from build123d import *

# Parameters (mm, degrees)
SKETCH2_W           = 508
SKETCH2_H           = 965.2
BOSS_EXTRUDE1_DEPTH = 152.4
FILLET1_R           = 15.24
FILLET2_R           = 15.24
SKETCH5_R           = 50.8
CUT_EXTRUDE1_DEPTH  = 718.072186045


with BuildPart() as part:
    # Sketch2 → Boss-Extrude1 (new body)
    with BuildSketch(Plane(origin=(0, 0, 0), x_dir=(1, 0, 0), z_dir=(0, 1, 0))):
        Rectangle(SKETCH2_W, SKETCH2_H)
    extrude(amount=BOSS_EXTRUDE1_DEPTH)

    # Fillet1
    fillet1_edges = [part.edges().sort_by_distance(p)[0] for p in [
        (-254, 152.4, 0),
        (0, 152.4, 482.6),
        (254, 152.4, 0),
        (0, 152.4, -482.6),
    ]]
    fillet(fillet1_edges, radius=FILLET1_R)

    # Fillet2
    # the kernel refuses this fillet: 15.24 mm, written as the material it takes off along each edge
    with BuildSketch(Plane(origin=(238.76, 137.16, -467.36), x_dir=(1, 0, 0), z_dir=(0, 0, -1))) as fillet2_piece_1_section:
        Polygon((0, 0), (FILLET2_R, 0), (FILLET2_R, -FILLET2_R), (0, -FILLET2_R), align=None)
    fillet2_piece_1 = extrude(amount=FILLET2_R, mode=Mode.PRIVATE)
    fillet2_piece_1 = fillet2_piece_1 - Plane(origin=(238.76, 137.16, -467.36), x_dir=(-0.7071067811865475, -0.7071067811865475, 0), z_dir=(0, 0, -1)) * Sphere(FILLET2_R, mode=Mode.PRIVATE)
    add(fillet2_piece_1, mode=Mode.SUBTRACT)
    with BuildSketch(Plane(origin=(238.76, 137.16, 467.36), x_dir=(0, 0, 1), z_dir=(1, 0, 0))) as fillet2_piece_2_section:
        Polygon((0, 0), (FILLET2_R, 0), (FILLET2_R, -FILLET2_R), (0, -FILLET2_R), align=None)
    fillet2_piece_2 = extrude(amount=FILLET2_R, mode=Mode.PRIVATE)
    fillet2_piece_2 = fillet2_piece_2 - Plane(origin=(238.76, 137.16, 467.36), x_dir=(0, -0.7071067811865475, -0.7071067811865475), z_dir=(1, 0, 0)) * Sphere(FILLET2_R, mode=Mode.PRIVATE)
    add(fillet2_piece_2, mode=Mode.SUBTRACT)
    with BuildSketch(Plane(origin=(-238.76, 137.16, -467.36), x_dir=(-1, 0, 0), z_dir=(0, 0, -1))) as fillet2_piece_3_section:
        Polygon((0, 0), (FILLET2_R, 0), (FILLET2_R, FILLET2_R), (0, FILLET2_R), align=None)
    fillet2_piece_3 = extrude(amount=FILLET2_R, mode=Mode.PRIVATE)
    fillet2_piece_3 = fillet2_piece_3 - Plane(origin=(-238.76, 137.16, -467.36), x_dir=(0.7071067811865475, -0.7071067811865475, 0), z_dir=(0, 0, -1)) * Sphere(FILLET2_R, mode=Mode.PRIVATE)
    add(fillet2_piece_3, mode=Mode.SUBTRACT)
    with BuildSketch(Plane(origin=(-238.76, 137.16, 467.36), x_dir=(0, 0, 1), z_dir=(-1, 0, 0))) as fillet2_piece_4_section:
        Polygon((0, 0), (FILLET2_R, 0), (FILLET2_R, FILLET2_R), (0, FILLET2_R), align=None)
    fillet2_piece_4 = extrude(amount=FILLET2_R, mode=Mode.PRIVATE)
    fillet2_piece_4 = fillet2_piece_4 - Plane(origin=(-238.76, 137.16, 467.36), x_dir=(0, -0.7071067811865475, -0.7071067811865475), z_dir=(-1, 0, 0)) * Sphere(FILLET2_R, mode=Mode.PRIVATE)
    add(fillet2_piece_4, mode=Mode.SUBTRACT)
    with BuildSketch(Plane(origin=(-238.76, 15.24, 467.36), x_dir=(0, -1, 0), z_dir=(-1, 0, 0))) as fillet2_piece_5_section:
        Polygon((0, 0), (FILLET2_R, 0), (FILLET2_R, FILLET2_R), (0, FILLET2_R), align=None)
    fillet2_piece_5 = extrude(amount=FILLET2_R, mode=Mode.PRIVATE)
    fillet2_piece_5 = fillet2_piece_5 - Plane(origin=(-238.76, 15.24, 467.36), x_dir=(0, 0.7071067811865475, -0.7071067811865475), z_dir=(-1, 0, 0)) * Sphere(FILLET2_R, mode=Mode.PRIVATE)
    add(fillet2_piece_5, mode=Mode.SUBTRACT)
    with BuildSketch(Plane(origin=(-238.76, 15.24, -467.36), x_dir=(-1, 0, 0), z_dir=(0, 0, -1))) as fillet2_piece_6_section:
        Polygon((0, 0), (FILLET2_R, 0), (FILLET2_R, -FILLET2_R), (0, -FILLET2_R), align=None)
    fillet2_piece_6 = extrude(amount=FILLET2_R, mode=Mode.PRIVATE)
    fillet2_piece_6 = fillet2_piece_6 - Plane(origin=(-238.76, 15.24, -467.36), x_dir=(0.7071067811865475, 0.7071067811865475, 0), z_dir=(0, 0, -1)) * Sphere(FILLET2_R, mode=Mode.PRIVATE)
    add(fillet2_piece_6, mode=Mode.SUBTRACT)
    with BuildSketch(Plane(origin=(238.76, 15.24, 467.36), x_dir=(1, 0, 0), z_dir=(0, -1, 0))) as fillet2_piece_7_section:
        Polygon((0, 0), (FILLET2_R, 0), (FILLET2_R, FILLET2_R), (0, FILLET2_R), align=None)
    fillet2_piece_7 = extrude(amount=FILLET2_R, mode=Mode.PRIVATE)
    fillet2_piece_7 = fillet2_piece_7 - Plane(origin=(238.76, 15.24, 467.36), x_dir=(-0.7071067811865477, 0, -0.7071067811865474), z_dir=(0, -1, 0)) * Sphere(FILLET2_R, mode=Mode.PRIVATE)
    add(fillet2_piece_7, mode=Mode.SUBTRACT)
    with BuildSketch(Plane(origin=(238.76, 15.24, -467.36), x_dir=(0, -1, 0), z_dir=(0, 0, -1))) as fillet2_piece_8_section:
        Polygon((0, 0), (FILLET2_R, 0), (FILLET2_R, -FILLET2_R), (0, -FILLET2_R), align=None)
    fillet2_piece_8 = extrude(amount=FILLET2_R, mode=Mode.PRIVATE)
    fillet2_piece_8 = fillet2_piece_8 - Plane(origin=(238.76, 15.24, -467.36), x_dir=(-0.7071067811865475, 0.7071067811865475, 0), z_dir=(0, 0, -1)) * Sphere(FILLET2_R, mode=Mode.PRIVATE)
    add(fillet2_piece_8, mode=Mode.SUBTRACT)
    with BuildSketch(Plane(origin=(-254, 15.24, 482.6), x_dir=(0, 0, -1), z_dir=(0, 1, 0)), Plane(origin=(-254, 15.24, -482.6), x_dir=(1, 0, 0), z_dir=(0, 1, 0))) as fillet2_piece_9:
        with BuildLine():
            CenterArc((FILLET2_R, -FILLET2_R), FILLET2_R, 90, 90)
            Line((0, -FILLET2_R), (0, 0))
            Line((0, 0), (FILLET2_R, 0))
        make_face()
    extrude(amount=121.92, mode=Mode.SUBTRACT)
    with BuildSketch(Plane(origin=(254, 15.24, 482.6), x_dir=(0, 0, -1), z_dir=(0, 1, 0)), Plane(origin=(254, 15.24, -482.6), x_dir=(-1, 0, 0), z_dir=(0, 1, 0))) as fillet2_piece_10:
        with BuildLine():
            CenterArc((FILLET2_R, FILLET2_R), FILLET2_R, 180, 90)
            Line((0, FILLET2_R), (0, 0))
            Line((0, 0), (FILLET2_R, 0))
        make_face()
    extrude(amount=121.92, mode=Mode.SUBTRACT)
    with BuildSketch(Plane(origin=(238.76, 0, 482.6), x_dir=(0, 0, -1), z_dir=(-1, 0, 0))) as fillet2_piece_11:
        with BuildLine():
            CenterArc((FILLET2_R, -FILLET2_R), FILLET2_R, 90, 90)
            Line((0, -FILLET2_R), (0, 0))
            Line((0, 0), (FILLET2_R, 0))
        make_face()
    extrude(amount=477.52, mode=Mode.SUBTRACT)
    with BuildSketch(Plane(origin=(-254, 0, 467.36), x_dir=(0, 1, 0), z_dir=(0, 0, -1))) as fillet2_piece_12:
        with BuildLine():
            CenterArc((FILLET2_R, FILLET2_R), FILLET2_R, 180, 90)
            Line((0, FILLET2_R), (0, 0))
            Line((0, 0), (FILLET2_R, 0))
        make_face()
    extrude(amount=934.72, mode=Mode.SUBTRACT)
    with BuildSketch(Plane(origin=(-238.76, 0, -482.6), x_dir=(0, 1, 0), z_dir=(1, 0, 0))) as fillet2_piece_13:
        with BuildLine():
            CenterArc((FILLET2_R, FILLET2_R), FILLET2_R, 180, 90)
            Line((0, FILLET2_R), (0, 0))
            Line((0, 0), (FILLET2_R, 0))
        make_face()
    extrude(amount=477.52, mode=Mode.SUBTRACT)
    with BuildSketch(Plane(origin=(254, 0, -467.36), x_dir=(-1, 0, 0), z_dir=(0, 0, 1))) as fillet2_piece_14:
        with BuildLine():
            CenterArc((FILLET2_R, -FILLET2_R), FILLET2_R, 90, 90)
            Line((0, -FILLET2_R), (0, 0))
            Line((0, 0), (FILLET2_R, 0))
        make_face()
    extrude(amount=934.72, mode=Mode.SUBTRACT)

    # Sketch5 → Cut-Extrude1 (cut, through all)
    with BuildSketch(Plane.ZY.offset(254)):
        with Locations((-365.76, 76.2)):
            Circle(SKETCH5_R)
        with Locations(Location((365.76, 76.2, 0), (0, 0, 180))):
            Circle(SKETCH5_R)
    extrude(amount=-CUT_EXTRUDE1_DEPTH, mode=Mode.SUBTRACT)


solid = part.part
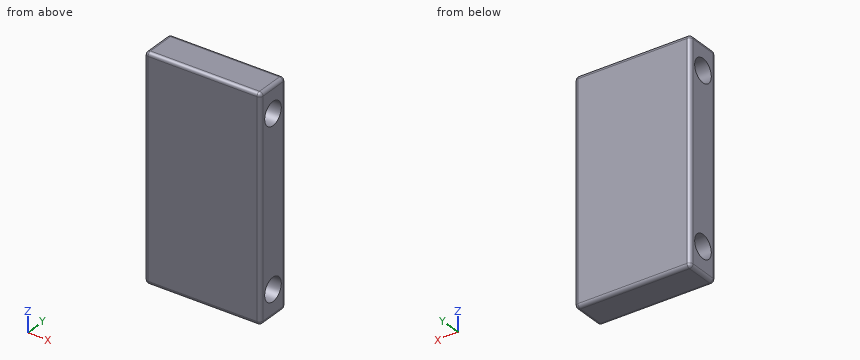
Design review of the part built by this model. Coordinates are the model's own, in mm. Give positions to 0.01 mm unless a question says otherwise; leave off trailing zeros. Order: outer loops, then holes, each group sorted by start corner. A loop starts at its lowest first (then second) coordinate and runs counter-clockwise, first axis right, second up.
1. Add section C-C, the plane y = 76.2. State the section outline as (x, z) points, then the cut area to 3 significant figures.
Solution:
outline: (-254, -467.36) arc R15.24 ccw to (-238.76, -482.6) - (238.76, -482.6) arc R15.24 ccw to (254, -467.36) - (254, -416.56) - (-254, -416.56) - close; (-254, -314.96) - (254, -314.96) - (254, 314.96) - (-254, 314.96) - close; (-254, 416.56) - (254, 416.56) - (254, 467.36) arc R15.24 ccw to (238.76, 482.6) - (-238.76, 482.6) arc R15.24 ccw to (-254, 467.36) - close
area: 387,000 mm2
2. To check wall thickness, follow L1, parallel to Z at x = -131, y = 76; L2, parallel to Y at x = -94, z = -365; L3, parallel to Z at x = 216.5, y = 69. State the ranges of each line that lie inside material, in increasing order.
Solution:
L1: z = -482.6 to -416.56, -314.96 to 314.96, 416.56 to 482.6
L2: y = 0 to 25.41, 126.99 to 152.4
L3: z = -482.6 to -416.05, -315.47 to 315.47, 416.05 to 482.6
3. Add section B-B, the plane x = -121. State the section outline as (y, z) points.
Solution:
outline: (0, -467.36) arc R15.24 ccw to (15.24, -482.6) - (137.16, -482.6) arc R15.24 ccw to (152.4, -467.36) - (152.4, 467.36) arc R15.24 ccw to (137.16, 482.6) - (15.24, 482.6) arc R15.24 ccw to (0, 467.36) - close; hole circle Ø101.6 at (76.2, -365.76); hole circle Ø101.6 at (76.2, 365.76)
4. Add section A-A, the plane z = 365.76. State the section outline as (x, y) points.
Solution:
outline: (-254, 15.24) arc R15.24 ccw to (-238.76, 0) - (238.76, 0) arc R15.24 ccw to (254, 15.24) - (254, 25.4) - (-254, 25.4) - close; (-254, 127) - (254, 127) - (254, 137.16) arc R15.24 ccw to (238.76, 152.4) - (-238.76, 152.4) arc R15.24 ccw to (-254, 137.16) - close
